Here's how the part is built. I have some questions about the finished solid (model axes, mm). Round coordinates to 2 decimals unless told otherwise and drop trailing zeros. Order: outer loops, then holes, each group sorted by start corner. A loop starts at its lowest first (then second) coordinate and runs counter-clockwise, first axis right, second up. Notation, with made-up numbers: (22.5, 8) -> (28.5, 8) arc R17 ccw to (28.5, 29) -> close; hole circle Ø11 at (74.5, 81). An arc over 180 degrees is marked (long way). Answer in a Markdown table with one row per item.
```python
from build123d import *

# Parameters (mm, degrees)
F1_DEPTH = 1270
F2_R     = 101.6
F3_DEPTH = 1270.001
F4_DEPTH = 25.4


with BuildPart() as f1:
    # F0 (on Top) → F1 (new body)
    with BuildSketch(Plane.XY):
        with BuildLine():
            ThreePointArc((152.4, 76.2), (-85.1941899427, 360.8883798855), (0, 0))
            Line((0, 0), (1016, 0))
            Line((1016, 0), (1016, 76.2))
            Line((1016, 76.2), (152.4, 76.2))
        make_face()
    extrude(amount=F1_DEPTH)

    # F2 (on face) → F3 (cut, through all)
    with BuildSketch(Plane.XY.offset(1270)):
        with Locations((0, 190.5)):
            Circle(F2_R)
    extrude(amount=-F3_DEPTH, mode=Mode.SUBTRACT)

    # F4 (add): a face of the model
    f4_faces = [f1.faces().sort_by_distance(p)[0] for p in [
        (508, 0, 635),
    ]]
    extrude(f4_faces, amount=F4_DEPTH)


solid = f1.part
```
1. Suppose I cut it at C-C on x = -27. Write out the boundary of the cut face in (y, z).
Numbers:
| item | result |
|---|---|
| outline | (1.92, 0) -> (92.55, 0) -> (92.55, 1270) -> (1.92, 1270) -> close; (288.45, 0) -> (379.08, 0) -> (379.08, 1270) -> (288.45, 1270) -> close |
2. Suppose I cut it at A-A on y = 190.5. Write out the boundary of the cut face in (x, z), then the cut area to 3 significant figures.
Numbers:
| item | result |
|---|---|
| outline | (-190.5, 0) -> (-101.6, 0) -> (-101.6, 1270) -> (-190.5, 1270) -> close; (101.6, 0) -> (190.5, 0) -> (190.5, 1270) -> (101.6, 1270) -> close |
| area | 226,000 mm2 |
3. We'd pull the mould along Z, two halves only. Please class faces 1 (the face through (270, 45, 1270)), 2 (the face through (270, 45, 0)), 3 (the face through (590, 76.2, 626)): released by +Z, released by -Z, zero draft, split by the parting line, or undercut.
Numbers:
| item | result |
|---|---|
| face 1 | released by +Z |
| face 2 | released by -Z |
| face 3 | zero draft |
4. Please list where these lines run through material, in increasing order: line 1 along Y through (x, z) = (455, 1067); line 2 along Y through (x, z) = (167, 1061.5); line 3 along X through (y, z) = (124, 1015.5).
Numbers:
| item | result |
|---|---|
| line 1 | y = -25.4 to 76.2 |
| line 2 | y = -25.4 to 76.2, 98.84 to 282.16 |
| line 3 | x = -178.52 to -76.81, 76.81 to 178.52 |
5. Suppose I cut it at D-D on x = 482. Write out the boundary of the cut face in (y, z), then the cut area to 3 significant figures.
Numbers:
| item | result |
|---|---|
| outline | (-25.4, 0) -> (76.2, 0) -> (76.2, 1270) -> (-25.4, 1270) -> close |
| area | 129,000 mm2 |
6. For pin 1 Ø8 at (y, z) = (240, 243) entering from -X; pin 2 Ø5 at (y, z) = (163.5, 1047) entering from -X; pin 3 Ø5 at (x, z) = (475, 196.5) entering from +Y, each with a flat end and sliding along its axis, tell me the tip position at first contact or that it passes through.
Numbers:
| item | result |
|---|---|
| pin 1 | stops at x = -184.99 |
| pin 2 | stops at x = -188.92 |
| pin 3 | stops at y = 76.2 |
7. Suppose I cut it at B-B on z = 222. Write out the boundary of the cut face in (x, y), then the cut area to 3 significant figures.
Numbers:
| item | result |
|---|---|
| outline | (0, -25.4) -> (1016, -25.4) -> (1016, 76.2) -> (152.4, 76.2) arc R190.5 ccw (long way) to (0, 0) -> close; hole circle Ø203.2 at (0, 190.5) |
| area | 177,000 mm2 |
